Could you check a few things on this model? Use its own coordinates, in mm. Face numbers are marked on the shaded views. A direction names the side the tool comes from. Round coordinates to 2 decimals unless told otherwise and drop trailing zeros. Write each loop counter-clockwise with the first axis right and the second up, starting at its lowest first coordinate (ties: lowest second). Pieces come first, ordered by that corner, then holes. Notation, with made-up numbers: (-24, 74) -> (2, 74) arc R22 ccw to (2, 102) -> close; hole circle Ø8 at (79.25, -2). An arc over 180 degrees is marked (long way). One line per question, with ' | ' between items. Start each with the question number.
1. Imagine slicing it at A-A, the plane z = 6.5. List the corners of the cut face in (x, y) for me.
2. For pin 1 Ø6 at (x, y) = (6.5, -4) entering from -Z; pin 2 Ø1 at (x, z) = (1.5, 4) entering from +Y; pin 3 Ø5 at (x, y) = (7, -3.5) entering from +Z, each with a flat end and sliding along its axis, tell me the tip position at first contact or that it passes through.
3. For the marked faces 1 and 2, which set-ups out of +Z, -Z, +X, -X, +Y, -Y let a thin tool reach every point of the face, with its end or its side?
4. If I drill on line 1 along Y through (x, z) = (0, -40.5); line 2 along Z through (x, y) = (1.75, 7.5); line 3 along Z through (x, y) = (3, 8.5), over which ranges is the centre line in solid material (lowest first)? Write a range as [from, to].
from build123d import *

# Parameters (mm, degrees)
F0_W     = 2.54
F0_H     = 69.85
F2_SIZE2 = 2.54
F2_SIZE  = 10.16
F3_R     = 5.08


# Not quite as in the source:
# - a fillet or chamfer that OpenCascade refuses, or shapes differently, is made with other operations: its cross-section is extruded or revolved along the edge and cut away or added


with BuildPart() as f1:
    # F0 (on Front) → F1 (revolve)
    with BuildSketch(Plane.XZ):
        Polygon((0, 14.605), (0, 12.7), (2.54, 12.7), (10.16, 12.7), (10.16, 14.605), align=None)
        with Locations((1.27, -22.225)):
            Rectangle(F0_W, F0_H)
    revolve(axis=Axis((0, 0, -22.225), (0, 0, -1)))

    # F2
    f2_edges = [f1.edges().sort_by_distance(p)[0] for p in [
        (-2.54, 0, -57.15),
    ]]
    f2_side = f1.faces().sort_by_distance((-2.54, 0, -22.225))[0]
    chamfer(f2_edges, length=F2_SIZE, length2=F2_SIZE2, reference=f2_side)

    # F3
    f3_edges = [f1.edges().sort_by_distance(p)[0] for p in [
        (-2.54, 0, 12.7),
    ]]
    fillet(f3_edges, radius=F3_R)

    # F4: fillet of radius 10.16 on 1 edges, made by hand

    # F4_s1 → F4_t2 (revolve, cut)
    with BuildSketch(Plane.XZ):
        with BuildLine():
            ThreePointArc((10.16, 12.7), (7.3479662746, 14.1170318444), (4.2371143013, 14.605))
            Line((4.2371143013, 14.605), (10.16, 14.605))
            Line((10.16, 14.605), (10.16, 12.7))
        make_face()
    revolve(axis=Axis((0, 0, 14.605), (0, 0, -1)), mode=Mode.SUBTRACT)


solid = f1.part
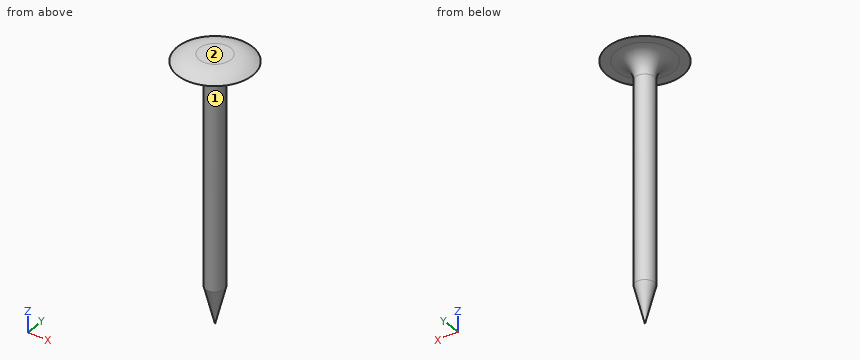
Geometry results:
1) outline: circle Ø5.08 at (0, 0)
2) pin 1: stops at z = 11.73 | pin 2: stops at y = 2.33 | pin 3: stops at z = 14.55
3) face 1: -Z | face 2: +Z, +X, -X, +Y, -Y
4) line 1: y = [-2.54, 2.54] | line 2: z = [12.7, 14] | line 3: z = [12.7, 13.41]
